```python
from build123d import *

# Parameters (mm, degrees)
BOSS_EXTRUDE1_DEPTH = 1219.2
FILLET1_R           = 0.254
SKETCH4_W           = 1905.2
SKETCH4_H           = 74.945320812
CUT_EXTRUDE1_DEPTH  = 60
SKETCH9_R           = 1.65
CUT_EXTRUDE5_DEPTH  = 60
SKETCH10_R          = 1.65
CUT_EXTRUDE6_DEPTH  = 60


with BuildPart() as part:
    # Sketch3 → Boss-Extrude1 (new, symmetric)
    with BuildSketch(Plane.XY):
        Polygon((1.5875, 25.4), (0, 25.4), (0, 0), (25.4, 0), (25.4, 1.5875), (1.5875, 1.5875), align=None)
    extrude(amount=BOSS_EXTRUDE1_DEPTH, both=True)

    # Fillet1
    fillet1_edges = [part.edges().sort_by_distance(p)[0] for p in [
        (1.5875, 1.5875, 0),
    ]]
    fillet(fillet1_edges, radius=FILLET1_R)

    # Sketch4 → Cut-Extrude1 (cut)
    with BuildSketch(Plane.ZY):
        with Locations((-266.6, 37.472660406)):
            Rectangle(SKETCH4_W, SKETCH4_H)
    extrude(amount=-CUT_EXTRUDE1_DEPTH, mode=Mode.SUBTRACT)

    # Sketch9 → Cut-Extrude5 (cut)
    with BuildSketch(Plane(origin=(1.5875, 0, 0), x_dir=(0, 0, -1), z_dir=(1, 0, 0))):
        with Locations((-1201.7375, 10.3759)):
            Circle(SKETCH9_R)
        with Locations((-703.4625, 10.3759)):
            Circle(SKETCH9_R)
        with Locations((-722.6, 13.49375)):
            Circle(SKETCH9_R)
        with Locations((-742.6, 13.49375)):
            Circle(SKETCH9_R)
        with Locations((-762.6, 13.49375)):
            Circle(SKETCH9_R)
        with Locations((-782.6, 13.49375)):
            Circle(SKETCH9_R)
        with Locations((-802.6, 13.49375)):
            Circle(SKETCH9_R)
        with Locations((-822.6, 13.49375)):
            Circle(SKETCH9_R)
        with Locations((-842.6, 13.49375)):
            Circle(SKETCH9_R)
        with Locations((-862.6, 13.49375)):
            Circle(SKETCH9_R)
        with Locations((-882.6, 13.49375)):
            Circle(SKETCH9_R)
        with Locations((-902.6, 13.49375)):
            Circle(SKETCH9_R)
        with Locations((-922.6, 13.49375)):
            Circle(SKETCH9_R)
        with Locations((-942.6, 13.49375)):
            Circle(SKETCH9_R)
        with Locations((-962.6, 13.49375)):
            Circle(SKETCH9_R)
        with Locations((-982.6, 13.49375)):
            Circle(SKETCH9_R)
        with Locations((-1002.6, 13.49375)):
            Circle(SKETCH9_R)
        with Locations((-1022.6, 13.49375)):
            Circle(SKETCH9_R)
        with Locations((-1042.6, 13.49375)):
            Circle(SKETCH9_R)
        with Locations((-1062.6, 13.49375)):
            Circle(SKETCH9_R)
        with Locations((-1082.6, 13.49375)):
            Circle(SKETCH9_R)
        with Locations((-1102.6, 13.49375)):
            Circle(SKETCH9_R)
        with Locations((-1122.6, 13.49375)):
            Circle(SKETCH9_R)
        with Locations((-1142.6, 13.49375)):
            Circle(SKETCH9_R)
        with Locations((-1162.6, 13.49375)):
            Circle(SKETCH9_R)
        with Locations((-1182.6, 13.49375)):
            Circle(SKETCH9_R)
    extrude(amount=-CUT_EXTRUDE5_DEPTH, mode=Mode.SUBTRACT)

    # Sketch10 → Cut-Extrude6 (cut)
    with BuildSketch(Plane(origin=(0, 1.5875, 0), x_dir=(1, 0, 0), z_dir=(0, 1, 0))):
        with Locations(Location((11.1125, -696.408204333, 0), (0, 0, 180))):
            Circle(SKETCH10_R)
        with Locations(Location((11.1125, -1208.791795667, 0), (0, 0, 180))):
            Circle(SKETCH10_R)
        with Locations(Location((13.49375, -1182.6, 0), (0, 0, 180))):
            Circle(SKETCH10_R)
        with Locations(Location((13.49375, -1162.6, 0), (0, 0, 180))):
            Circle(SKETCH10_R)
        with Locations(Location((13.49375, -1142.6, 0), (0, 0, 180))):
            Circle(SKETCH10_R)
        with Locations(Location((13.49375, -1122.6, 0), (0, 0, 180))):
            Circle(SKETCH10_R)
        with Locations(Location((13.49375, -1102.6, 0), (0, 0, 180))):
            Circle(SKETCH10_R)
        with Locations(Location((13.49375, -1082.6, 0), (0, 0, 180))):
            Circle(SKETCH10_R)
        with Locations(Location((13.49375, -1062.6, 0), (0, 0, 180))):
            Circle(SKETCH10_R)
        with Locations(Location((13.49375, -1042.6, 0), (0, 0, 180))):
            Circle(SKETCH10_R)
        with Locations(Location((13.49375, -1022.6, 0), (0, 0, 180))):
            Circle(SKETCH10_R)
        with Locations(Location((13.49375, -1002.6, 0), (0, 0, 180))):
            Circle(SKETCH10_R)
        with Locations(Location((13.49375, -982.6, 0), (0, 0, 180))):
            Circle(SKETCH10_R)
        with Locations(Location((13.49375, -962.6, 0), (0, 0, 180))):
            Circle(SKETCH10_R)
        with Locations(Location((13.49375, -942.6, 0), (0, 0, 180))):
            Circle(SKETCH10_R)
        with Locations(Location((13.49375, -922.6, 0), (0, 0, 180))):
            Circle(SKETCH10_R)
        with Locations(Location((13.49375, -902.6, 0), (0, 0, 180))):
            Circle(SKETCH10_R)
        with Locations(Location((13.49375, -882.6, 0), (0, 0, 180))):
            Circle(SKETCH10_R)
        with Locations(Location((13.49375, -862.6, 0), (0, 0, 180))):
            Circle(SKETCH10_R)
        with Locations(Location((13.49375, -842.6, 0), (0, 0, 180))):
            Circle(SKETCH10_R)
        with Locations(Location((13.49375, -822.6, 0), (0, 0, 180))):
            Circle(SKETCH10_R)
        with Locations(Location((13.49375, -802.6, 0), (0, 0, 180))):
            Circle(SKETCH10_R)
        with Locations(Location((13.49375, -782.6, 0), (0, 0, 180))):
            Circle(SKETCH10_R)
        with Locations(Location((13.49375, -762.6, 0), (0, 0, 180))):
            Circle(SKETCH10_R)
        with Locations(Location((13.49375, -742.6, 0), (0, 0, 180))):
            Circle(SKETCH10_R)
        with Locations(Location((13.49375, -722.6, 0), (0, 0, 180))):
            Circle(SKETCH10_R)
    extrude(amount=-CUT_EXTRUDE6_DEPTH, mode=Mode.SUBTRACT)


solid = part.part
```
Geometry check sheet. Reference: the model listing, model coordinates, mm. A direction names the side the tool comes from. Coordinates: 2 decimals unless noted, no trailing zeros. Order: outer loops, then holes, each group sorted by start corner. A loop starts at its lowest first (then second) coordinate and runs counter-clockwise, first axis right, second up.
Item 1: Section check B-B (y = 21.5). Enter the section's corners in (x, z), plus the area to 3 significant figures.
Item 2: Scan lines: line 1 along X through (y, z) = (1.25, 1162.6); line 2 along Y through (x, z) = (6.5, 1094.5). Record each from-to range of solid material in increasing order.
Item 3: Section check A-A (z = 994.5). Enter the section's corners in (x, y).
Item 4: Depth check by flat-ended pin: pin 1 (5.5 mm diameter, centred on x = 13.49, z = 1162.6, fed in from +Y); pin 2 (10 mm diameter, centred on y = 12, z = 1127.5, fed in from +X); pin 3 (2 mm diameter, centred on x = 13.49, z = 882.6, fed in from +Y); pin 4 (5.5 mm diameter, centred on x = 13.49, z = 862.6, fed in from -Y). Enter the tip coordinate at first touch or a pass-through.
Item 5: Tool access check on faces 1 (the flat face through (13, 0, 956)), 2 (the flat face through (14, 1.588, 956)). Record the directions out of +Z, -Z, +X, -X, +Y, -Y that give a thin tool (end or side, any length) a straight path to the whole face; none if there is none.
Check sheet entries:
1. outline: (0, 686) - (1.59, 686) - (1.59, 1219.2) - (0, 1219.2) - close
1. area: 846 mm2
2. line 1: x = 0 to 11.84, 15.14 to 25.4
2. line 2: y = 0 to 1.59
3. outline: (0, 0) - (25.4, 0) - (25.4, 1.59) - (1.84, 1.59) arc R0.25 cw to (1.59, 1.84) - (1.59, 25.4) - (0, 25.4) - close
4. pin 1: stops at y = 1.59
4. pin 2: stops at x = 1.59
4. pin 3: passes through
4. pin 4: stops at y = 0
5. face 1: +Z, -Z, +X, -X, -Y
5. face 2: +Z, -Z, +X, +Y
